Autodesk Inventor part; units mm, degrees
ref_plane "YZ Plane" through (0, 0, 0) normal (1, 0, 0) x (0, 1, 0)
ref_plane "XZ Plane" through (0, 0, 0) normal (0, 1, 0) x (-1, 0, 0)
ref_plane "XY Plane" through (0, 0, 0) normal (0, 0, 1) x (1, 0, 0)
sketch "Sketch1" plane through (0, 0, 0) normal (0, 1, 0) x (-1, 0, 0)
  line L0 (0, 0) -> (119.38, 0)
  line L1 (119.38, -9.525) -> (9.525, -9.525)
  line L2 (0, -9.525) -> (0, 0)
  arc A0 (0, -9.525) -> (9.525, -9.525) centre (4.7625, -10.16) ccw
  arc A1 (119.38, -9.525) -> (119.38, 0) centre (117.4254, -4.7625) ccw
  circle A2 centre (117.4254, -4.7625) radius 2.2479
  circle A3 centre (101.4234, -4.7625) radius 2.2479
  circle A4 centre (83.872, -4.7625) radius 1.9685
  circle A5 centre (74.093, -4.7625) radius 1.9685
  circle A6 centre (64.314, -4.7625) radius 1.9685
  circle A7 centre (54.535, -4.7625) radius 1.9685
  circle A8 centre (44.756, -4.7625) radius 1.9685
  circle A9 centre (34.977, -4.7625) radius 1.9685
  circle A10 centre (25.198, -4.7625) radius 1.9685
  circle A11 centre (15.419, -4.7625) radius 1.9685
  dimension "d9" = 9.525
  dimension "d10" = 119.38
  dimension "d11" = 4.4958
  dimension "d12" = 4.4958
  dimension "d13" = 16.002
  dimension "d14" = 3.937
  dimension "d15" = 17.5514
  dimension "d18" = 9.779
extrude "Extrusion1" add sketch "Sketch1" along normal blind 3.175
sketch "Sketch2" plane through (0, 3.175, 0) normal (0, 1, 0) x (1, 0, 0)
  circle A0 centre (-34.977, 4.7625) radius 1.9685 construction
  arc A1 (0, 9.525) -> (-9.525, 9.525) centre (-4.7625, 10.16) ccw construction
  line L0 (0, 0) -> (-6.35, 0)
  line L1 (-6.35, 0) -> (-6.35, 9.525)
  line L2 (-9.525, 9.525) -> (-6.35, 9.525)
  line L3 (0, 9.525) -> (0, 0)
  line L4 (-119.38, 0) -> (0, 0)
  line L5 (0, 0) -> (0, 9.525)
  arc A2 (0, 9.525) -> (-9.525, 9.525) centre (-4.7625, 10.16) ccw
  point P0 (-4.7625, 4.7625)
  dimension "d27" = 0
  dimension "d28" = 6.35
  dimension "d32" = 0
extrude "Extrusion2" add sketch "Sketch2" along normal blind 9.525
fillet "Fillet2" radius 3.175 1 edges at (0, 6.35, 0)
properties part number "Rear Collector Arm"
Here's how the part is built. I have some questions about the finished solid (model axes, mm). A direction names the side the tool comes from. Give positions to 0.01 mm unless a question says otherwise; leave off trailing zeros. Write each loop counter-clockwise with the first axis right and the second up, starting at its lowest first coordinate (ties: lowest second). Pieces come first, ordered by that corner, then holes. Notation, with made-up numbers: (50.25, 20) -> (67.25, 20) arc R33 ccw to (67.25, 48) -> close; hole circle Ø11 at (58.5, 32.25). An arc over 180 degrees is marked (long way). Write each question's results on one line, items separated by ' | '.
Item 1: If I drill on L1, parallel to X at y = 10.5, z = -6; L2, parallel to Y at x = -114, z = -1.5 (3 decimals); L3, parallel to X at y = 11.25, z = -10.5, over which ranges is the centre line in solid material (lowest first)?
Output:
L1: x = -6.35 to 0 | L2: y = 0 to 3.175 | L3: x = -9.56 to 0.03
Item 2: On a 3-axis mill with a long thin cutter (end or side, diameter ignored), from which of +Z, -Z, +X, -X, +Y, -Y can I reach the whole of each face in a straight line? I mean faces 1 (the face through (-57, 3, 0)), 2 (the face through (-65, 2, -9.525)), 3 (the face through (-6.35, 8, -5)). Say none if no direction works.
Output:
face 1: +Z, +X, -X, +Y, -Y | face 2: -Z, -X, +Y, -Y | face 3: +Z, -X, +Y
Item 3: Suppose I cut it at C-C on z = -8.5. Write out the boundary of the cut face in (x, y) (3 decimals), plus the area to 3 significant figures.
Output:
outline: (-120.966, 0) -> (0, 0) -> (0, 12.7) -> (-6.35, 12.7) -> (-6.35, 3.175) -> (-120.966, 3.175) -> close | area: 445 mm^2
Item 4: For pin 1 Ø4.5 at (x, z) = (-15.42, -4.76) entering from +Y (3 decimals); pin 2 Ø1 at (y, z) = (11, -2.5) entering from +X; pin 3 Ø2.5 at (x, y) = (-74, 1) entering from -Z (3 decimals); pin 4 Ø8 at (x, z) = (-49, -9.5) entering from -Y, each with a flat end and sliding along its axis, tell me the tip position at first contact or that it passes through.
Output:
pin 1: stops at y = 3.175 | pin 2: stops at x = 0 | pin 3: stops at z = -9.525 | pin 4: stops at y = 0
Item 5: We'd pull the mould along Z, two halves only. Please class faces 4 (the face through (-85.69, 1.57, -4.01)), 5 (the face through (-122.573, 1.565, -4.677)), 6 (the face through (-4, 12.7, -8)): pulls with the +Z half, pulls with the -Z half, needs draft (parallel to the pull), parting line crosses it, or undercut.
Output:
face 4: undercut | face 5: parting line crosses it | face 6: needs draft
Item 6: Suppose I cut it at A-A on x = -65. Write out the boundary of the cut face in (y, z) (3 decimals), plus the area to 3 significant figures.
Output:
outline: (0, -9.525) -> (3.175, -9.525) -> (3.175, -6.608) -> (0, -6.608) -> close; (0, -2.917) -> (3.175, -2.917) -> (3.175, 0) -> (0, 0) -> close | area: 18.5 mm^2
